Build history of the part. All positions in model axes, mm. A direction names the side the tool comes from. Coordinates: 2 decimals unless noted, no trailing zeros. Loops run counter-clockwise (first coordinate to the right, second up) from the corner with the lowest first, then second, coordinate; pieces in that order, holes last.
(1) Tool access for faces 5 (the face through (-19, 7, 41.1)), 6 (the face through (4, 0, 154.8)), 7 (the face through (4, 9, -48)), 8 (the face through (-9.76, -2.17, -48.76)), 9 (the face through (-0.1, 17.5, 61.1)): list every direction of +Z, -Z, +X, -X, +Y, -Y with a clear straight run to the whole face (end or side of a thin tool).
(2) Slice it at A-A (z = 109.5). Give the cut face in (x, y).
(3) Two-plate mould, pull along Y, no slides. Class faces 1 (the face through (0, 6.5, 142)), 2 (the face through (-0.35, 0.078, 138.774)), 3 (the face through (-17.847, -2.343, 87.054)), 4 (the face through (5, -16, 36.1)): pulls with the +Y half, pulls with the -Y half, needs draft (parallel to the pull), parting line crosses it, or undercut.
(4) Flat gauge pins, fed straight in: P1, Ø12, axis at x = 17, z = 101, coming from the +Y side; P2, Ø1.2, axis at y = 17.5, z = 50.5, coming from the -X side; P3, Ø8, axis at x = -2.5, y = 10, coming from the -Z side; P4, Ø6, axis at y = -0.5, z = 37.5, coming from the -X side. Where does each tip first touch, or does it go through?
(5) Wall check: L1, parallel to Y at x = 0, z = 143.75; L2, parallel to X at y = 0, z = 144; L3, parallel to Z at x = -7.5, y = 18.5. Give the ranges that are in metal, low to high.
(6) Slice it at B-B (z = 88). Give the cut face in (x, y).
Autodesk Inventor part; units mm, degrees
ref_plane "Wellennuttiefe_Arbeitsebene_2" through (0, 6.5, 126.35) normal (0, 1, 0) x (-1, 0, 0)
ref_plane "YZ Plane" through (0, 0, 0) normal (1, 0, 0) x (0, 1, 0)
ref_plane "XY Plane" through (0, 0, 0) normal (0, 0, 1) x (1, 0, 0)
sketch "Skizze1" plane through (0, 0, 0) normal (1, 0, 0) x (0, 1, 0)
  line L0 (0, 154.8) -> (9, 154.8)
  line L1 (9, 154.8) -> (10, 153.8)
  line L2 (10, 153.8) -> (10, 98.9)
  line L3 (18, 75.9) -> (20, 73.9)
  line L4 (20, 73.9) -> (20, 65.3)
  line L5 (20, 61.3) -> (20, 41.1)
  line L6 (20, 41.1) -> (23.5, 41.1)
  line L7 (23.5, 41.1) -> (23.5, 36.1)
  line L8 (23.5, 36.1) -> (16.5, 36.1)
  line L9 (16.5, 36.1) -> (16.5, -13.8)
  line L10 (10, -15.8) -> (10, -46.7)
  line L11 (10, -46.7) -> (9.5, -46.7)
  line L12 (9.5, -46.7) -> (9.5, -48)
  line L13 (9.5, -48) -> (10, -48)
  line L14 (10, -48) -> (10, -49.5)
  line L15 (10, -49.5) -> (9.5, -50)
  line L16 (9.5, -50) -> (0, -50)
  line L17 (0, -50) -> (0, 154.8)
  line L18 (14.5, -15.8) -> (10, -15.8)
  line L19 (16.5, -13.8) -> (14.5, -15.8)
  line L20 (0, 195.76) -> (0, -90.96) construction
  line L21 (-4.7, 0) -> (28.2, 0) construction
  line L22 (10, 98.9) -> (0, 98.9) construction
  line L23 (10, -15.8) -> (0, -15.8) construction
  line L24 (10, -46.7) -> (0, -46.7) construction
  line L25 (17, 98.9) -> (10, 98.9)
  line L26 (18, 75.9) -> (18, 97.9)
  line L27 (18, 97.9) -> (17, 98.9)
  line L28 (10, 129.8) -> (0, 129.8) construction
  circle A0 centre (20, 63.3) radius 2 construction
  line L29 (20, 65.3) -> (19.0799, 64.3799)
  line L30 (19.0799, 64.3799) -> (19.0799, 62.2201)
  line L31 (19.0799, 62.2201) -> (20, 61.3)
  line L32 (20, 63.3) -> (19.0799, 63.3) construction
  point P0 (0, 0)
  point P1 (18, 98.9)
  dimension "d4" = 45
  dimension "d6" = 1.3
  dimension "d9" = 23.5
  dimension "d11" = 5
  dimension "d19" = 45
  dimension "d20" = 2
  dimension "d21" = 2
  dimension "d22" = 1
  dimension "d34" = 0
  dimension "d35" = 50
  dimension "d36" = 45
  dimension "d87" = 114.7
  dimension "d88" = 0
  dimension "d89" = 30.9
  dimension "d90" = 19
  dimension "d91" = 20
  dimension "d119" = 20
  dimension "d120" = 1.5
  dimension "d122" = 1
  dimension "d123" = 1
  dimension "d124" = 33
  dimension "d125" = 40
  dimension "d126" = 30.9
  dimension "d127" = 25
  dimension "d135" = 78.9
  dimension "d139" = 91.5
  dimension "d140" = 113.7
  dimension "d141" = 22.2
  dimension "d142" = 45
  dimension "d143" = 45
  dimension "d144" = 38.1598
  dimension "d145" = 8.6
revolve "Umdrehung1" add sketch "Skizze1" angle 360 about axis through (0, 0, -50) along (0, 0, 1)
ref_plane "Wellennuttiefe_Arbeitsebene" through (0, 15, 51.2) normal (0, 1, 0) x (-1, 0, 0)
ref_plane "Arbeitsebene1" through (0, 20, 51.2) normal (0, 1, 0) x (-1, 0, 0)
sketch "Skizze2" plane through (0, 20, 51.2) normal (0, 1, 0) x (-1, 0, 0)
  line L0 (0, 9.9) -> (0, -10.1) construction
  line L1 (6, 3.9) -> (6, -4.1)
  line L2 (-6, -4.1) -> (-6, 3.9)
  arc A0 (6, 3.9) -> (-6, 3.9) centre (0, 3.9) ccw
  arc A1 (-6, -4.1) -> (6, -4.1) centre (0, -4.1) ccw
  line L3 (-23.5, -10.1) -> (23.5, -10.1) construction
  line L4 (0, 144.56) -> (0, -142.16) construction
  point P0 (0, -51.2)
  point P1 (0, -0.1)
  dimension "d29" = 20
  dimension "d30" = 12
extrude "Passfeder_Ausnahme" cut sketch "Skizze2" against normal up to surface (5 mm away)
thread "Gewinde1"
ref_plane "Arbeitsebene5" through (0, 10, 126.35) normal (0, 1, 0) x (-1, 0, 0)
sketch "Skizze7" plane through (0, 10, 126.35) normal (0, 1, 0) x (-1, 0, 0)
  line L0 (-10, -27.45) -> (10, -27.45) construction
  line L1 (10, 3.45) -> (-10, 3.45) construction
  line L2 (-10, -27.45) -> (10, -27.45) construction
  line L3 (0, -27.45) -> (0, 3.45) construction
  line L4 (10, 27.45) -> (10, -27.45) construction
  line L5 (-10, 27.45) -> (-10, -27.45) construction
  line L6 (0, 10.95) -> (0, 20.95) construction
  line L7 (3, 10.95) -> (3, 20.95)
  line L8 (-3, 20.95) -> (-3, 10.95)
  arc A0 (-3, 10.95) -> (3, 10.95) centre (0, 10.95) ccw
  arc A1 (3, 20.95) -> (-3, 20.95) centre (0, 20.95) ccw
  line L9 (0, 7.95) -> (3, 7.95) construction
  line L10 (-9, 28.45) -> (9, 28.45) construction
  line L11 (-17, -27.45) -> (17, -27.45) construction
  line L12 (0, 28.45) -> (0, 3.45) construction
  point P0 (0, -126.35)
  point P1 (0, 15.95)
  point P2 (0, 23.95)
  dimension "d100" = 30.9
  dimension "d101" = 6
  dimension "d102" = 16
  dimension "Flansch_Max_Connector_Lenght" = 25
ref_plane "Wellennuttiefe_Arbeitsebene_2" through (0, 6.5, 126.35) normal (0, 1, 0) x (-1, 0, 0)
extrude "PassfederNut_HeadSide" cut sketch "Skizze7" against normal up to surface (3.5 mm away)
sketch "Skizze9" plane through (0, 0, 154.8) normal (0, 0, 1) x (1, 0, 0)
  circle A0 centre (0, 0) radius 9 construction
  point P0 (0, 0)
hole "Bohrung1" at (0, 0, 154.8) direction (0, 0, -1) diameter 4.134 depth 15 tip angle 118
chamfer "Fase4" distance 1.5 angle 45 1 edges at (0, 2.067, 154.8)
equation "\"d6\" = Sprengring_NutBreite"
equation "\"d87\" = -MainAxis_Bearing_Fix2ScrewLimit_Dist + Gestell_Lager_Distanz - MainAxis_Bearing_Fix2Limit_Dist"
equation "\"d89\" = MainAxis_Bearing_Fix2Limit_Dist + MainAxis_Bearing_Fix2ScrewLimit_Dist"
equation "\"d90\" = Sprengring_NutDurchmesser"
equation "\"d91\" = P204_ShaftDiameter"
equation "\"d119\" = P204_ShaftDiameter"
equation "\"d29\" = Passfeder_length"
equation "\"d100\" = MainAxis_Bearing_Fix2ScrewLimit_Dist + MainAxis_Bearing_Fix2Limit_Dist"
equation "\"Wellennuttiefe_20\" = 3.5"
equation "\"Nabennuttiefe_20\" = 2.8"
equation "\"Sprengring_NutBreite\" = 1.3"
equation "\"Sprengring_NutDurchmesser\" = 19"
equation "\"Nabennuttiefe_40\" = 3.3"
equation "\"Wellennuttiefe_40\" = 5"
equation "\"Passfeder_Width_20\" = 6"
equation "\"Passfeder_Width_40\" = 12"
properties part number "Welle" material "Edelstahl"
Response values:
1. face 5: +Z
1. face 6: +Z, +X, -X, +Y, -Y
1. face 7: none
1. face 8: -Z
1. face 9: +Y
2. outline: circle Ø20 at (0, 0)
3. face 1: pulls with the +Y half
3. face 2: undercut
3. face 3: parting line crosses it
3. face 4: needs draft
4. P1: stops at y = 13.54
4. P2: stops at x = -10.7
4. P3: stops at z = -50
4. P4: stops at x = -23.5
5. L1: y = -10 to -2.07, 2.07 to 6.5
5. L2: x = -10 to -2.07, 2.07 to 10
5. L3: z = 36.1 to 61.34, 65.26 to 73.94
6. outline: circle Ø36 at (0, 0)
